```python
from build123d import *

# Parameters (mm, degrees)
ESQUISSE1_W             = 240
ESQUISSE1_H             = 50
BOSS_EXTRU_1_DEPTH      = 5
ESQUISSE2_W             = 240
ESQUISSE2_H             = 5
BOSS_EXTRU_2_DEPTH      = 50
ESQUISSE4_R             = 5
ENL_V_MAT_EXTRU_1_DEPTH = 5
ESQUISSE5_W             = 240
ESQUISSE5_H             = 5
BOSS_EXTRU_3_DEPTH      = 10


with BuildPart() as part:
    # Esquisse1 → Boss.-Extru.1 (new body)
    with BuildSketch(Plane.XY):
        with Locations((-120, 25)):
            Rectangle(ESQUISSE1_W, ESQUISSE1_H)
    extrude(amount=BOSS_EXTRU_1_DEPTH)

    # Esquisse2 → Boss.-Extru.2 (add)
    with BuildSketch(Plane(origin=(0, 50, 0), x_dir=(1, 0, 0), z_dir=(0, 1, 0))):
        with Locations((-120, -2.5)):
            Rectangle(ESQUISSE2_W, ESQUISSE2_H)
    extrude(amount=BOSS_EXTRU_2_DEPTH)

    # Esquisse4 → Enlèv. mat.-Extru.1 (cut)
    with BuildSketch(Plane.XY.offset(5)):
        with Locations((-92, 82.7)):
            Circle(ESQUISSE4_R)
    extrude(amount=-ENL_V_MAT_EXTRU_1_DEPTH, mode=Mode.SUBTRACT)

    # Esquisse5 → Boss.-Extru.3 (add)
    with BuildSketch(Plane(origin=(0, 100, 0), x_dir=(1, 0, 0), z_dir=(0, 1, 0))):
        with Locations((-120, -2.5)):
            Rectangle(ESQUISSE5_W, ESQUISSE5_H)
    extrude(amount=BOSS_EXTRU_3_DEPTH)


solid = part.part
```
CAD build for the part. Positions are in the model's coordinates, mm. Coordinates: 2 decimals unless noted, no trailing zeros. Write each loop counter-clockwise with the first axis right and the second up, starting at its lowest first coordinate (ties: lowest second). Pieces come first, ordered by that corner, then holes. Notation, with made-up numbers: (44.5, 36) -> (67.5, 36) arc R28 ccw to (67.5, 67) -> close; hole circle Ø2 at (-34, -20.75). An arc over 180 degrees is marked (long way). Return JSON: item names as keys, results as strings. Group by question number.
Q1. Flat gauge pin, fed straight in: pin 1 (3 mm diameter, centred on y = 98.5, z = 3, fed in from +X). Where does the tip first touch, or does it go through?
Q2. Drill centre line: line 1 (Y direction, x = -92, z = 3.8). Where is it in solid material? Low to high.
Q3. Pull direction Y, two halves, no side cores. Call faces 1 (the face through (-89.693, 78.264, 2.535)), 2 (the face through (-122, 110, 2)), 3 (the face through (-240, 54, 3)): released by +Y, released by -Y, zero draft, split by the parting line, or undercut.
Q4. Cut at A-A, the plane y = 82.7. Give the cut face in (x, z), then the cut area to 3 significant figures.
Q5. Cut at B-B, the plane x = -92. Give the cut face in (y, z).
Returned:
{
 "1": {"pin 1": "stops at x = 0"},
 "2": {"line 1": "y = 0 to 77.7, 87.7 to 110"},
 "3": {"face 1": "undercut", "face 2": "released by +Y", "face 3": "zero draft"},
 "4": {"outline": "(-240, 0) -> (-97, 0) -> (-97, 5) -> (-240, 5) -> close; (-87, 0) -> (0, 0) -> (0, 5) -> (-87, 5) -> close", "area": "1,150 mm2"},
 "5": {"outline": "(0, 0) -> (77.7, 0) -> (77.7, 5) -> (0, 5) -> close; (87.7, 0) -> (110, 0) -> (110, 5) -> (87.7, 5) -> close"}
}
